```python
from build123d import *

# Parameters (mm, degrees)
SKETCH2_OUTSIDE_W  = 58.616
SKETCH2_OUTSIDE_H  = 58.616
CUT_EXTRUDE1_DEPTH = 110.75
SKETCH4_OUTSIDE_W  = 58.616
SKETCH4_OUTSIDE_H  = 58.616
CUT_EXTRUDE3_DEPTH = 3.75
SKETCH5_OUTSIDE_W  = 58.616
SKETCH5_OUTSIDE_H  = 58.616
CUT_EXTRUDE4_DEPTH = 3.5


with BuildPart() as part:
    # Sketch1 → Revolve1 (revolve)
    with BuildSketch(Plane.XY, mode=Mode.PRIVATE) as revolve1_sk:
        with BuildLine():
            Line((0, 0), (0, 15.375))
            Line((0, 15.375), (1.2, 15.375))
            Line((1.2, 15.375), (1.2, 9.5))
            ThreePointArc((1.2, 9.5), (1.492893219, 8.792893219), (2.2, 8.5))
            Line((2.2, 8.5), (17.112879499, 8.5))
            ThreePointArc((17.112879499, 8.5), (21.455437353, 12.535653753), (27.2, 14))
            Line((27.2, 14), (82.2, 14))
            Line((82.2, 14), (85.7, 7.5))
            Line((85.7, 7.5), (89.2, 14))
            Line((89.2, 14), (111.95, 14))
            Line((111.95, 14), (111.95, 14.5))
            Line((111.95, 14.5), (113.15, 14.5))
            Line((113.15, 14.5), (113.15, 7.75))
            Line((113.15, 7.75), (116.9, 7.75))
            Line((116.9, 7.75), (116.9, 10.5))
            Line((116.9, 10.5), (118.3, 10.5))
            Line((118.3, 10.5), (121.8, 0))
            Line((121.8, 0), (0, 0))
        make_face()
    revolve(revolve1_sk.sketch.rotate(Axis((121.8, 0, 0), (-1, 0, 0)), 90), axis=Axis((121.8, 0, 0), (-1, 0, 0)))

    # Sketch2 outside → Cut-Extrude1 (cut)
    with BuildSketch(Plane(origin=(1.2, 0, 0), x_dir=(0, 0, -1), z_dir=(1, 0, 0))):
        Rectangle(SKETCH2_OUTSIDE_W, SKETCH2_OUTSIDE_H)
        with BuildLine():
            Line((-0.6, 15.363288222), (-0.6, 0.6))
            Line((-0.6, 0.6), (-15.363288222, 0.6))
            ThreePointArc((-15.363288222, 0.6), (-15.375, 0), (-15.363288222, -0.6))
            Line((-15.363288222, -0.6), (-0.6, -0.6))
            Line((-0.6, -0.6), (-0.6, -15.363288222))
            ThreePointArc((-0.6, -15.363288222), (0, -15.375), (0.6, -15.363288222))
            Line((0.6, -15.363288222), (0.6, -0.6))
            Line((0.6, -0.6), (15.363288222, -0.6))
            ThreePointArc((15.363288222, -0.6), (15.375, 0), (15.363288222, 0.6))
            Line((15.363288222, 0.6), (0.6, 0.6))
            Line((0.6, 0.6), (0.6, 15.363288222))
            ThreePointArc((0.6, 15.363288222), (0, 15.375), (-0.6, 15.363288222))
        make_face(mode=Mode.SUBTRACT)
    extrude(amount=CUT_EXTRUDE1_DEPTH, mode=Mode.SUBTRACT)

    # Sketch4 outside → Cut-Extrude3 (cut)
    with BuildSketch(Plane(origin=(113.15, 0, 0), x_dir=(0, 0, -1), z_dir=(1, 0, 0))):
        Rectangle(SKETCH4_OUTSIDE_W, SKETCH4_OUTSIDE_H)
        with BuildLine():
            Line((0.6, 0.6), (0.6, 15.363288222))
            ThreePointArc((0.6, 15.363288222), (0, 15.375), (-0.6, 15.363288222))
            Line((-0.6, 15.363288222), (-0.6, 0.6))
            Line((-0.6, 0.6), (-15.363288222, 0.6))
            ThreePointArc((-15.363288222, 0.6), (-15.375, 0), (-15.363288222, -0.6))
            Line((-15.363288222, -0.6), (-0.6, -0.6))
            Line((-0.6, -0.6), (-0.6, -15.363288222))
            ThreePointArc((-0.6, -15.363288222), (0, -15.375), (0.6, -15.363288222))
            Line((0.6, -15.363288222), (0.6, -0.6))
            Line((0.6, -0.6), (15.363288222, -0.6))
            ThreePointArc((15.363288222, -0.6), (15.375, 0), (15.363288222, 0.6))
            Line((15.363288222, 0.6), (0.6, 0.6))
        make_face(mode=Mode.SUBTRACT)
    extrude(amount=CUT_EXTRUDE3_DEPTH, mode=Mode.SUBTRACT)

    # Sketch5 outside → Cut-Extrude4 (cut)
    with BuildSketch(Plane(origin=(121.8, 0, 0), x_dir=(0, 0, -1), z_dir=(1, 0, 0))):
        Rectangle(SKETCH5_OUTSIDE_W, SKETCH5_OUTSIDE_H)
        with BuildLine():
            Line((0.6, 0.6), (0.6, 9.856755298))
            ThreePointArc((0.6, 9.856755298), (0, 9.875), (-0.6, 9.856755298))
            Line((-0.6, 9.856755298), (-0.6, 0.6))
            Line((-0.6, 0.6), (-9.856755298, 0.6))
            ThreePointArc((-9.856755298, 0.6), (-9.875, 0), (-9.856755298, -0.6))
            Line((-9.856755298, -0.6), (-0.6, -0.6))
            Line((-0.6, -0.6), (-0.6, -9.856755298))
            ThreePointArc((-0.6, -9.856755298), (0, -9.875), (0.6, -9.856755298))
            Line((0.6, -9.856755298), (0.6, -0.6))
            Line((0.6, -0.6), (9.856755298, -0.6))
            ThreePointArc((9.856755298, -0.6), (9.875, 0), (9.856755298, 0.6))
            Line((9.856755298, 0.6), (0.6, 0.6))
        make_face(mode=Mode.SUBTRACT)
    extrude(amount=-CUT_EXTRUDE4_DEPTH, mode=Mode.SUBTRACT)


solid = part.part
```
Read the model definition and answer for the solid it produces. Units are mm, in the model's axes. A direction names the side the tool comes from. Give positions to 0.01 mm unless a question says otherwise; leave off trailing zeros. Loops run counter-clockwise (first coordinate to the right, second up) from the corner with the lowest first, then second, coordinate; pieces in that order, holes last.
Item 1: The mould has two halves that part along X. Classify faces 5 (the flat face through (120, 4, -0.6)), 6 (the conical face through (87.474, -10.795, -0.012)), 7 (the conical face through (121.625, 0.229, 0.473)), 8 (the flat face through (115, 0.6, 4)): released by +X, released by -X, zero draft, split by the parting line, or undercut.
Item 2: Find the intervals of material crossed by line 1 along X through (y, z) = (2.5, -9); line 2 along X through (y, z) = (-3, 14); line 3 along Y through (x, z) = (7, 5.5), in increasing order.
Item 3: The part is cut by section B-B (z = -12). Give the number of separate pieces and of enclosed holes in the cut face, and give its area (3 significant figures).
Item 4: The part is cut by section A-A (x = 110.5). Write down the section's boundary in (y, z), and give its area (3 significant figures).
Item 5: Each of these flat-tipped pins is pushed along its axis until it touches: pin 1 Ø4 at (x, y) = (57, 8) entering from +Z; pin 2 Ø1.9 at (x, y) = (114, -4) entering from -Z; pin 3 Ø10 at (x, y) = (27.5, 9.5) entering from -Z. Where does it stop, or does it pass through?
Item 6: For faces 1 (the flat face through (116.9, 2, 2)), 2 (the flat face through (115, 0.6, -4)), 3 (the flat face through (56, 7, 0.6)), 4 (the flat face through (115, -4, -0.6)), determine the directions among +Z, -Z, +X, -X, +Y, -Y from which every point of the face is accessible in a straight line to the end or side of a thin tool.
Taken from the geometry:
1. face 5: zero draft
1. face 6: undercut
1. face 7: released by +X
1. face 8: undercut
2. line 1: x = 0 to 1.2, 111.95 to 113.15, 116.9 to 118.3
2. line 2: x = 0 to 1.2, 111.95 to 113.15
2. line 3: y = -0.6 to 0.6
3. separate pieces: 3
3. enclosed holes: 0
3. area: 146 mm2
4. outline: (-13.99, -0.6) - (-0.6, -0.6) - (-0.6, -13.99) arc R14 ccw to (0.6, -13.99) - (0.6, -0.6) - (13.99, -0.6) arc R14 ccw to (13.99, 0.6) - (0.6, 0.6) - (0.6, 13.99) arc R14 ccw to (-0.6, 13.99) - (-0.6, 0.6) - (-13.99, 0.6) arc R14 ccw to start
4. area: 65.7 mm2
5. pin 1: stops at z = 0.6
5. pin 2: stops at z = -14.05
5. pin 3: stops at z = -0.6
6. face 1: none
6. face 2: -Z, +Y
6. face 3: +Z, +Y
6. face 4: -Z, -Y
